Source: three-view drawing plus pictorial views. Frame: mm from the lowest corner of the part. Give positions to 0.01 mm unless a question says otherwise; leave off trailing zeros. Order: outer loops, then holes, each group sorted by start corner. A loop starts at its lowest first (then second) coordinate and runs counter-clockwise, first axis right, second up.
1) First-contact query: P1, Ø4, axis at x = 71.87, z = 31.75, coming from the +Y side; P2, Ø7, axis at x = 57.15, z = 60.325, coming from the +Y side (3 decimals); P3, Ø1.6, axis at x = 18.5, y = 2, coming from the -Z side. Flat tips, straight axial feed; report the tip coordinate or a pass-through.
2) Section B-B, the plane x = 71.87. Return loops of the section in (y, z) (3 decimals), plus the area to 3 significant figures.
3) Material intervals for line 1 (X direction, y = 1, z = 66.04) (3 decimals); line 2 (Z direction, x = 38.1, y = 1.8) (3 decimals); line 3 (Z direction, x = 71.87, y = 1.25), sorted ascending.
4) Section D-D, the plane z = 101.6. Return loops of the section in (x, y) (3 decimals), plus the area to 3 significant figures.
5) Section A-A, the plane z = 31.75. Return loops of the section in (x, y) (3 decimals), plus the area to 3 significant figures.
6) Section C-C, the plane y = 1.45. Give the number of separate pieces and of enclosed holes in the cut face, plus the area to 3 significant figures.
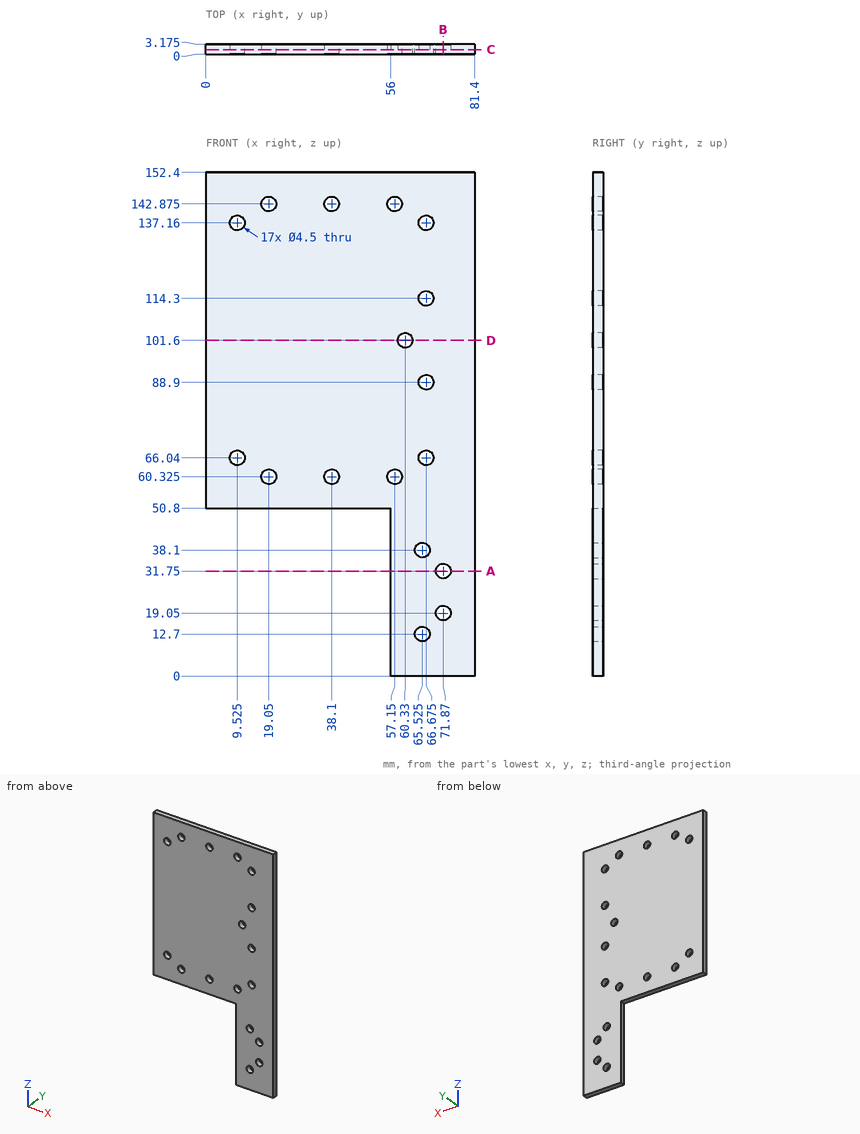
From the geometry:
1. P1: passes through
1. P2: stops at y = 3.175
1. P3: stops at z = 50.8
2. outline: (0, 0) - (3.175, 0) - (3.175, 16.8) - (0, 16.8) - close; (0, 21.3) - (3.175, 21.3) - (3.175, 29.5) - (0, 29.5) - close; (0, 34) - (3.175, 34) - (3.175, 152.4) - (0, 152.4) - close
2. area: 455 mm2
3. line 1: x = 0 to 7.275, 11.775 to 64.425, 68.925 to 81.4
3. line 2: z = 50.8 to 58.075, 62.575 to 140.625, 145.125 to 152.4
3. line 3: z = 0 to 16.8, 21.3 to 29.5, 34 to 152.4
4. outline: (0, 0) - (58.08, 0) - (58.08, 3.175) - (0, 3.175) - close; (62.58, 0) - (81.4, 0) - (81.4, 3.175) - (62.58, 3.175) - close
4. area: 244 mm2
5. outline: (56, 0) - (69.62, 0) - (69.62, 3.175) - (56, 3.175) - close; (74.12, 0) - (81.4, 0) - (81.4, 3.175) - (74.12, 3.175) - close
5. area: 66.4 mm2
6. separate pieces: 1
6. enclosed holes: 17
6. area: 9,290 mm2
